Here's the drawing with two shaded views (mm, measured from the low corner). I have some questions. Give positions to 0.01 mm unless a question says otherwise; leave off trailing zeros. Loops run counter-clockwise (first coordinate to the right, second up) from the corner with the lowest first, then second, coordinate; pieces in that order, holes last. Notation, with made-up numbers: (78, -4) - (122, -4) arc R32 cw to (122, 26) - close; hole circle Ø8 at (83, -21). An arc over 180 degrees is marked (long way). Answer as a JSON object with one key per item and string values. Group by question number.
Item 1: Suppose I cut it at C-C on y = 41.5. Write out the boundary of the cut face in (x, z), and give its area (3 significant figures).
Item 2: Please list where these lines run through material, in increasing order: L1, parallel to Y at x = 10, z = 2.95; L2, parallel to X at y = 66, z = 1.95; L3, parallel to X at y = 43.5, z = 2.5.
Item 3: Suppose I cut it at A-A on z = 3.2. Write out the boundary of the cut face in (x, y), and give its area (3 significant figures).
Item 4: Will this pin go through, and if not, where does the flat tip stop? pin 1 (2 mm diameter, centred on y = 39.5, z = 4, fed in from +X).
Item 5: Suppose I cut it at B-B on x = 10. Write out the boundary of the cut face in (y, z), and give its area (3 significant figures).
Item 6: Thinking about a two-plate mould opening in Z: for the marked faces 1 and 2, which applies, pulls with the +Z half, pulls with the -Z half, needs draft (parallel to the pull), parting line crosses it, or undercut?
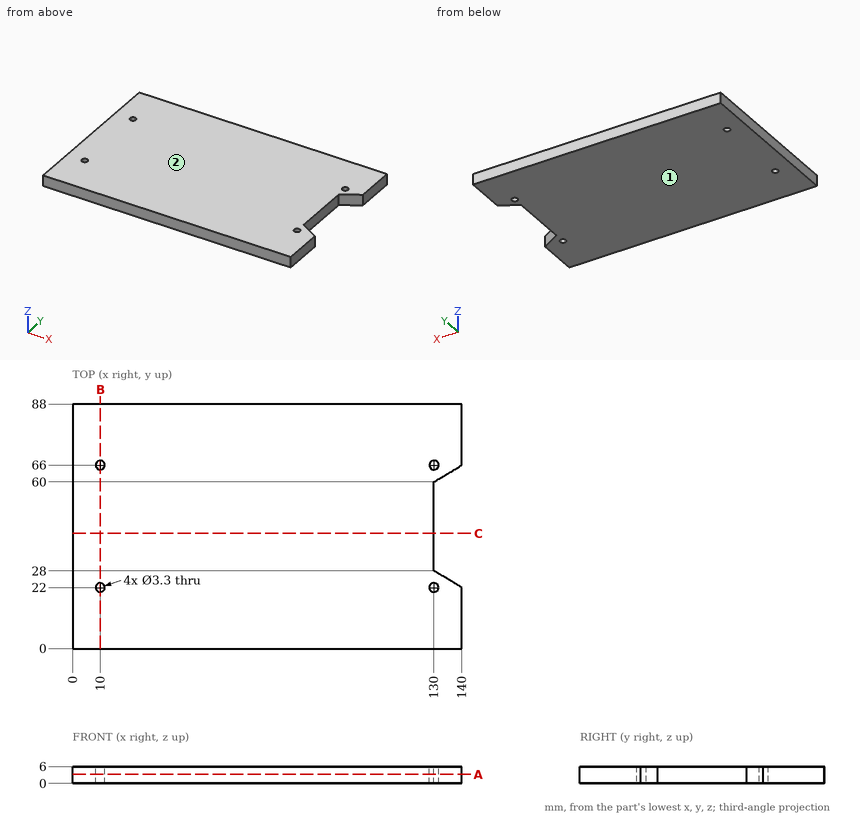
Worked out:
{
 "1": {"outline": "(0, 0) - (130, 0) - (130, 6) - (0, 6) - close", "area": "780 mm2"},
 "2": {"L1": "y = 0 to 20.35, 23.65 to 64.35, 67.65 to 88", "L2": "x = 0 to 8.35, 11.65 to 128.35, 131.65 to 140", "L3": "x = 0 to 130"},
 "3": {"outline": "(0, 0) - (140, 0) - (140, 22) - (130, 28) - (130, 60) - (140, 66) - (140, 88) - (0, 88) - close; hole circle Ø3.3 at (10, 22); hole circle Ø3.3 at (10, 66); hole circle Ø3.3 at (130, 22); hole circle Ø3.3 at (130, 66)", "area": "11,900 mm2"},
 "4": {"pin 1": "stops at x = 130"},
 "5": {"outline": "(0, 0) - (20.35, 0) - (20.35, 6) - (0, 6) - close; (23.65, 0) - (64.35, 0) - (64.35, 6) - (23.65, 6) - close; (67.65, 0) - (88, 0) - (88, 6) - (67.65, 6) - close", "area": "488 mm2"},
 "6": {"face 1": "pulls with the -Z half", "face 2": "pulls with the +Z half"}
}
